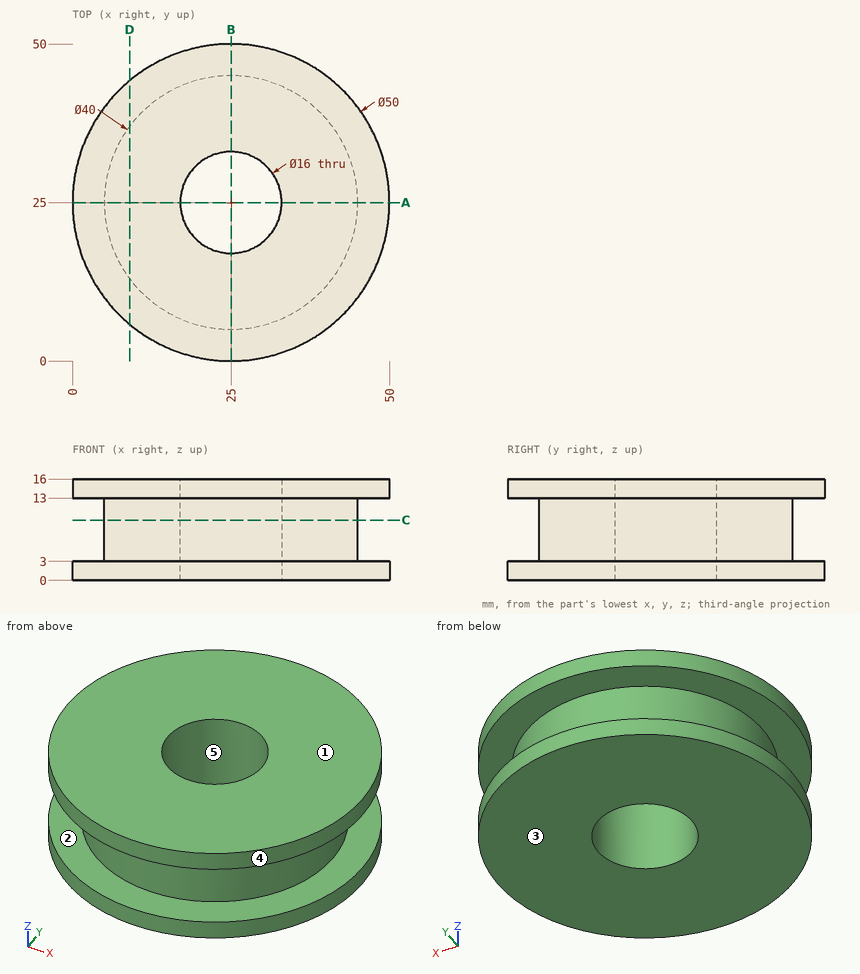
Print and shaded views of the part. All mm, measured from the part's lowest x, y and z. A direction names the side the tool comes from. Coordinates: 2 decimals unless noted, no trailing zeros. Order: outer loops, then holes, each group sorted by start corner. A loop starts at its lowest first (then second) coordinate and runs counter-clockwise, first axis right, second up. Notation, with made-up numbers: (-15, 42.25) - (15, 42.25) arc R17 ccw to (15, 66.25) - close; hole circle Ø11 at (-12, 22.25). An arc over 180 degrees is marked (long way). Put each result on its own line as item: value.
1. Tool access for the marked faces 1 and 2: list every direction of +Z, -Z, +X, -X, +Y, -Y with a clear straight run to the whole face (end or side of a thin tool).
Answer sheet:
face 1: +Z, +X, -X, +Y, -Y
face 2: none
2. Probe line 1 along Z through (x, y) = (5.5, 15); line 2 along Y through (x, z) = (25, 4.25); line 3 along Y through (x, z) = (26.5, 5.75). List the from-to ranges inside material, lowest first. Write a range as [from, to].
Answer sheet:
line 1: z = [0, 3], [13, 16]
line 2: y = [5, 17], [33, 45]
line 3: y = [5.06, 17.14], [32.86, 44.94]
3. Saw through at C-C (z = 9.5). Write the cut outline in (x, y).
Answer sheet:
outline: circle Ø40 at (25, 25); hole circle Ø16 at (25, 25)
4. Saw through at D-D (x = 9). Write the cut outline in (y, z).
Answer sheet:
outline: (5.79, 0) - (44.21, 0) - (44.21, 3) - (37, 3) - (37, 13) - (44.21, 13) - (44.21, 16) - (5.79, 16) - (5.79, 13) - (13, 13) - (13, 3) - (5.79, 3) - close
5. Drop flat-ended pins along their axis: P1, Ø8, axis at y = 43.5, z = 4.5, coming from the +X side; P2, Ø8, axis at y = 20.5, z = 8, coming from the +X side; P3, Ø6, axis at x = 25, z = 14, coming from the +Y side. Give the stop position or say it passes through.
Answer sheet:
P1: stops at x = 45.15
P2: stops at x = 44.99
P3: stops at y = 50
6. Saw through at A-A (y = 25). Write the cut outline in (x, z), and give its area (3 significant figures).
Answer sheet:
outline: (0, 0) - (17, 0) - (17, 16) - (0, 16) - (0, 13) - (5, 13) - (5, 3) - (0, 3) - close; (33, 0) - (50, 0) - (50, 3) - (45, 3) - (45, 13) - (50, 13) - (50, 16) - (33, 16) - close
area: 444 mm^2
7. Pull direction X, two halves, no side cores. Call the marked faces 3, 4 and 5: pulls with the +X half, pulls with the -X half, needs draft (parallel to the pull), parting line crosses it, or undercut.
Answer sheet:
face 3: needs draft
face 4: parting line crosses it
face 5: undercut
